from build123d import *

# Parameters (mm, degrees)
SKETCH1_R               = 1.143
BOSS_EXTRUDE1_DEPTH     = 1.5
CROQUIS1_W              = 16
CROQUIS1_H              = 16
SALIENTE_EXTRUIR1_DEPTH = 1
CROQUIS2_R              = 0.5
SALIENTE_EXTRUIR2_DEPTH = 79
SALIENTE_EXTRUIR3_DEPTH = 5.5
CORTAR_EXTRUIR1_DEPTH   = 95.596612016


with BuildPart() as part:
    # Sketch1 → Boss-Extrude1 (new body)
    with BuildSketch(Plane.XY.offset(3.527777778)):
        with BuildLine():
            Line((-11.43, 22.9), (-11.43, -22.9))
            ThreePointArc((-11.43, -22.9), (-10.697766953, -24.667766953), (-8.93, -25.4))
            Line((-8.93, -25.4), (8.93, -25.4))
            ThreePointArc((8.93, -25.4), (10.697766953, -24.667766953), (11.43, -22.9))
            Line((11.43, -22.9), (11.43, 22.9))
            ThreePointArc((11.43, 22.9), (10.697766953, 24.667766953), (8.93, 25.4))
            Line((8.93, 25.4), (-8.93, 25.4))
            ThreePointArc((-8.93, 25.4), (-10.697766953, 24.667766953), (-11.43, 22.9))
        make_face()
        with Locations(Location((9.525, 22.86, 0), (0, 0, 180))):
            Circle(SKETCH1_R, mode=Mode.SUBTRACT)
        with Locations(Location((-9.525, 22.86, 0), (0, 0, 180))):
            Circle(SKETCH1_R, mode=Mode.SUBTRACT)
        with Locations(Location((-9.525, -22.86, 0), (0, 0, 180))):
            Circle(SKETCH1_R, mode=Mode.SUBTRACT)
        with Locations(Location((9.525, -22.86, 0), (0, 0, 180))):
            Circle(SKETCH1_R, mode=Mode.SUBTRACT)
    extrude(amount=-BOSS_EXTRUDE1_DEPTH)

    # Croquis1 → Saliente-Extruir1 (add)
    with BuildSketch(Plane.XY.offset(3.527777778)):
        with Locations((-0.07, 13.4)):
            Rectangle(CROQUIS1_W, CROQUIS1_H)
    extrude(amount=SALIENTE_EXTRUIR1_DEPTH)

    # Croquis2 → Saliente-Extruir2 (add)
    with BuildSketch(Plane.XY.offset(3.527777778)):
        with Locations((6.43, 24.4)):
            Circle(CROQUIS2_R)
    extrude(amount=SALIENTE_EXTRUIR2_DEPTH)

    # Croquis3 → Saliente-Extruir3 (add)
    with BuildSketch(Plane.XY.offset(3.527777778)):
        Polygon((-11.43, -12.4), (-3.43, -12.4), (-3.43, -13.4), (-5.43, -13.4), (-5.43, -18.4), (-3.43, -18.4), (-3.43, -19.4), (-11.43, -19.4), align=None)
    extrude(amount=SALIENTE_EXTRUIR3_DEPTH)

    # Croquis4 → Cortar-Extruir1 (cut, through all)
    with BuildSketch(Plane.XZ.offset(19.4)):
        Polygon((-5.43, 9.027777778), (-5.43, 7.527777778), (-3.43, 6.027777778), (-3.43, 9.027777778), align=None)
    extrude(amount=-CORTAR_EXTRUIR1_DEPTH, mode=Mode.SUBTRACT)


solid = part.part
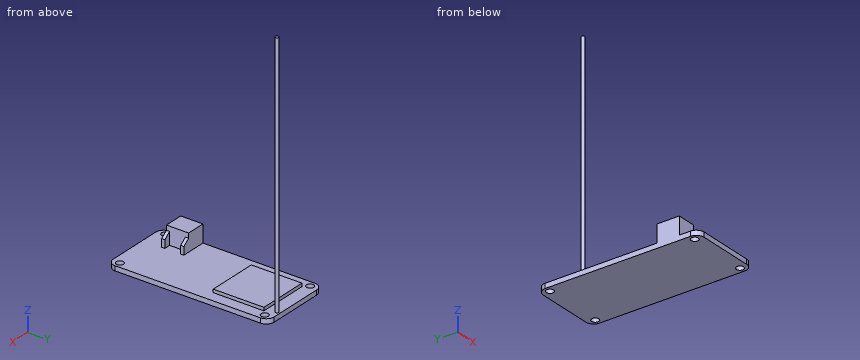
Input: part model. Units: mm. Frame: model coordinates. Give positions to 0.01 mm unless a question says otherwise; leave off trailing zeros. Order: outer loops, then holes, each group sorted by start corner. A loop starts at its lowest first (then second) coordinate and runs counter-clockwise, first axis right, second up. Notation, with made-up numbers: (-10.75, -1) - (-2.75, -1) arc R30 ccw to (-2.75, 24) - close; hole circle Ø9 at (37.25, 39.5). An arc over 180 degrees is marked (long way). Write each question's results on one line, items separated by ' | '.
Item 1: Section B-B (y = 19.5). Return loops of the section in (x, z).
A:
outline: (-11.43, 2.03) - (11.43, 2.03) - (11.43, 3.53) - (7.93, 3.53) - (7.93, 4.53) - (-8.07, 4.53) - (-8.07, 3.53) - (-11.43, 3.53) - close
Item 2: Contact query for flat-ended pins moving along their axis: pin 1 Ø6.5 at (x, y) = (-8, -17) entering from +Z; pin 2 Ø3 at (x, y) = (-9.525, -22.86) entering from +Z; pin 3 Ø6 at (y, z) = (-14.5, 6) entering from +X; pin 4 Ø1.6 at (x, z) = (-9.5, 5) entering from +Y. Output: stop coordinate, or through.
A:
pin 1: stops at z = 9.03 | pin 2: stops at z = 3.53 | pin 3: stops at x = 11.43 | pin 4: stops at y = -12.4
Item 3: Material intervals for line 1 along X through (y, z) = (-22.86, 3.1); line 2 along Z through (x, y) = (7, 4); line 3 along Z through (x, y) = (7.25, 6.5), sorted ascending.
A:
line 1: x = -11.43 to -10.67, -8.38 to 8.38, 10.67 to 11.43 | line 2: z = 2.03 to 3.53 | line 3: z = 2.03 to 4.53
Item 4: Section C-C (z = 30). Return loops of the section in (x, y).
A:
outline: circle Ø1 at (6.43, 24.4)
Item 5: Section A-A (x = -6.5). Return loops of the section in (y, z), and give its area (3 significant figures).
A:
outline: (-25.4, 2.03) - (25.4, 2.03) - (25.4, 3.53) - (21.4, 3.53) - (21.4, 4.53) - (5.4, 4.53) - (5.4, 3.53) - (-12.4, 3.53) - (-12.4, 9.03) - (-19.4, 9.03) - (-19.4, 3.53) - (-25.4, 3.53) - close | area: 131 mm^2
Item 6: Section D-D (x = 3.25). Return loops of the section in (y, z), and give its area (3 significant figures).
A:
outline: (-25.4, 2.03) - (25.4, 2.03) - (25.4, 3.53) - (21.4, 3.53) - (21.4, 4.53) - (5.4, 4.53) - (5.4, 3.53) - (-25.4, 3.53) - close | area: 92.2 mm^2
